from build123d import *

# Parameters (mm, degrees)
SKETCH1_R           = 1.524
BOSS_EXTRUDE1_DEPTH = 1.5875
SKETCH8_R           = 3.7465
SKETCH8_R_2         = 1.9685
BOSS_EXTRUDE6_DEPTH = 1.5875


with BuildPart() as part:
    # Sketch1 → Boss-Extrude1 (new body)
    with BuildSketch(Plane.XY):
        with BuildLine():
            Line((-301.9473, 133.57775), (-305.87795, 129.6471))
            Line((-305.87795, 129.6471), (-314.0123, 129.6471))
            Line((-314.0123, 129.6471), (-314.0123, 113.6451))
            Line((-314.0123, 113.6451), (-305.87795, 113.6451))
            Line((-305.87795, 113.6451), (-301.9473, 109.71445))
            Line((-301.9473, 109.71445), (-301.9473, 91.6317))
            ThreePointArc((-301.9473, 91.6317), (-303.063223164, 88.937623164), (-305.7573, 87.8217))
            Line((-305.7573, 87.8217), (-315.9973, 91.1883))
            Line((-315.9973, 91.1883), (-368.3165, 91.1883))
            Line((-368.3165, 91.1883), (-378.5565, 87.8217))
            Line((-378.5565, 87.8217), (-397.2472, 87.8217))
            ThreePointArc((-397.2472, 87.8217), (-399.951018769, 88.947400452), (-401.0571, 91.659304166))
            Line((-401.0571, 91.659304166), (-401.0571, 95.6449))
            Line((-401.0571, 95.6449), (-399.1521, 95.6449))
            Line((-399.1521, 95.6449), (-399.1521, 148.341))
            Line((-399.1521, 148.341), (-401.0571, 148.341))
            Line((-401.0571, 148.341), (-401.0571, 150.956597849))
            ThreePointArc((-401.0571, 150.956597849), (-399.946077222, 153.659592612), (-397.247125, 154.7804))
            Line((-397.247125, 154.7804), (-305.7573, 154.7804))
            ThreePointArc((-305.7573, 154.7804), (-303.063223164, 153.664476836), (-301.9473, 150.9704))
            Line((-301.9473, 150.9704), (-301.9473, 133.57775))
        make_face()
        with Locations((-305.7573, 150.9704)):
            Circle(SKETCH1_R, mode=Mode.SUBTRACT)
        with Locations((-397.247125, 150.9704)):
            Circle(SKETCH1_R, mode=Mode.SUBTRACT)
        with Locations((-397.2472, 91.6317)):
            Circle(SKETCH1_R, mode=Mode.SUBTRACT)
        with Locations((-305.7573, 91.6317)):
            Circle(SKETCH1_R, mode=Mode.SUBTRACT)
    extrude(amount=BOSS_EXTRUDE1_DEPTH)

    # Sketch8 → Boss-Extrude6 (add)
    with BuildSketch(Plane.XY.offset(1.5875)):
        with BuildLine():
            ThreePointArc((-379.068128555, 158.80105), (-382.814628555, 155.05455), (-386.561128555, 158.80105))
            Line((-386.561128555, 158.80105), (-386.561128555, 154.7804))
            Line((-386.561128555, 154.7804), (-379.068128555, 154.7804))
            Line((-379.068128555, 154.7804), (-379.068128555, 158.80105))
        make_face()
        with Locations((-382.814628555, 158.80105)):
            Circle(SKETCH8_R)
        with Locations((-382.814628555, 158.80105)):
            Circle(SKETCH8_R_2, mode=Mode.SUBTRACT)
        with BuildLine():
            Line((-311.561128555, 158.80105), (-311.561128555, 154.7804))
            Line((-311.561128555, 154.7804), (-305.7573, 154.7804))
            ThreePointArc((-305.7573, 154.7804), (-304.889939249, 154.680357591), (-304.068128555, 154.385484162))
            Line((-304.068128555, 154.385484162), (-304.068128555, 158.80105))
            ThreePointArc((-304.068128555, 158.80105), (-307.814628555, 155.05455), (-311.561128555, 158.80105))
        make_face()
        with Locations((-307.814628555, 158.80105)):
            Circle(SKETCH8_R)
        with Locations((-307.814628555, 158.80105)):
            Circle(SKETCH8_R_2, mode=Mode.SUBTRACT)
        with BuildLine():
            Line((-311.561128555, 89.729821994), (-311.561128555, 83.80105))
            ThreePointArc((-311.561128555, 83.80105), (-307.814628555, 87.54755), (-304.068128555, 83.80105))
            Line((-304.068128555, 83.80105), (-304.068128555, 88.216615838))
            ThreePointArc((-304.068128555, 88.216615838), (-304.889939249, 87.921742409), (-305.7573, 87.8217))
            Line((-305.7573, 87.8217), (-311.561128555, 89.729821994))
        make_face()
        with Locations((-307.814628555, 83.80105)):
            Circle(SKETCH8_R)
        with Locations((-307.814628555, 83.80105)):
            Circle(SKETCH8_R_2, mode=Mode.SUBTRACT)
        with BuildLine():
            ThreePointArc((-386.561128555, 83.80105), (-382.814628555, 87.54755), (-379.068128555, 83.80105))
            Line((-379.068128555, 83.80105), (-379.068128555, 87.8217))
            Line((-379.068128555, 87.8217), (-386.561128555, 87.8217))
            Line((-386.561128555, 87.8217), (-386.561128555, 83.80105))
        make_face()
        with Locations((-382.814628555, 83.80105)):
            Circle(SKETCH8_R)
        with Locations((-382.814628555, 83.80105)):
            Circle(SKETCH8_R_2, mode=Mode.SUBTRACT)
    extrude(amount=-BOSS_EXTRUDE6_DEPTH)


solid = part.part
Read the model definition and answer for the solid it produces. Units are mm, in the model's axes. A direction names the side the tool comes from. Give positions to 0.01 mm unless a question says otherwise; leave off trailing zeros. Write each loop counter-clockwise with the first axis right and the second up, starting at its lowest first coordinate (ties: lowest second). Pieces come first, ordered by that corner, then holes. Notation, with made-up numbers: (-36.5, 31) -> (-31.5, 31) arc R30 cw to (-31.5, 66) -> close; hole circle Ø11 at (35, 3). An arc over 180 degrees is marked (long way). Answer as a JSON object with one key per item and string values. Group by question number.
1) A tool of negligible diameter and unlimited length cuts with its end or side. For faces 1 (the flat face through (-303.94, 111.707, 0.783)), 2 (the flat face through (-352, 122, 0)), 3 (the flat face through (-373.36, 89.53, 0.78)), from which of +Z, -Z, +X, -X, +Y, -Y can it reach the whole face along a straight path? Write none if from no direction.
2) Find section C-C (x = -324.5). Write down the section's boundary in (y, z), and give its area (3 significant figures).
3) Find section B-B (y = 117.5). Write down the section's boundary in (x, z).
4) Each of these flat-tipped pins is pushed along its axis until it touches: P1, Ø0.5, axis at y = 119.5, z = 1, coming from the +X side; P2, Ø0.8, axis at y = 157, z = 0.5, coming from the +X side; P3, Ø0.8, axis at x = -339, z = 0.5, coming from the -Y side. Where does it stop, or does it pass through?
5) The mould has two halves that part along Y. Classify faces 4 (the cylindrical face through (-395.84, 150.39, 0.78)), 5 (the cylindrical face through (-302.54, 153.01, 0.78)), 6 (the cylindrical face through (-307.897, 80.055, 0.805)): +Y half, -Y half, draft (parallel to the pull), parting line (faces both ways), or undercut.
6) Consider L1, parallel to X at y = 158.5, z = 0.6; L2, parallel to Y at x = -309.5, z = 0.6; L3, parallel to X at y = 92.5, z = 0.7. Determine where each line is inside the solid, lowest interval first. Write a range as from..to.
7) Find section A-A (z = 0.4). Count the separate pieces of the cut face and the enclosed holes in it, and give its area (3 significant figures).
Values follow:
{
 "1": {"face 1": "+Z, -Z, +X", "face 2": "-Z, +X, -X, +Y, -Y", "face 3": "+Z, -Z, -Y"},
 "2": {"outline": "(91.19, 0) -> (154.78, 0) -> (154.78, 1.59) -> (91.19, 1.59) -> close", "area": "101 mm2"},
 "3": {"outline": "(-399.15, 0) -> (-314.01, 0) -> (-314.01, 1.59) -> (-399.15, 1.59) -> close"},
 "4": {"P1": "stops at x = -314.01", "P2": "stops at x = -304.07", "P3": "stops at y = 91.19"},
 "5": {"face 4": "undercut", "face 5": "+Y half", "face 6": "-Y half"},
 "6": {"L1": "x = -386.56..-384.76, -380.87..-379.07, -311.56..-309.76, -305.87..-304.07", "L2": "y = 80.46..82.78, 84.82..113.65, 129.65..157.78, 159.82..162.15", "L3": "x = -401.06..-398.5, -395.99..-307.01, -304.5..-301.95"},
 "7": {"separate pieces": "1", "enclosed holes": "8", "area": "6,240 mm2"}
}
